Design review of the part built by this model. Coordinates are the model's own, in mm. A direction names the side the tool comes from. Coordinates: 2 decimals unless noted, no trailing zeros. Loops run counter-clockwise (first coordinate to the right, second up) from the corner with the lowest first, then second, coordinate; pieces in that order, holes last. Notation, with made-up numbers: (10, -0.75) -> (61, -0.75) arc R22 ccw to (61, 18.25) -> close; hole circle Ø11 at (-17, 78.5). An arc over 180 degrees is marked (long way). Answer in a Markdown table with one row per item.
```python
from build123d import *

# Parameters (mm, degrees)
F1_DEPTH = 628.65
F2_R     = 4.76249
F4_DEPTH = 25.4


# Not quite as in the source:
# - a fillet or chamfer is up to 0.001 mm smaller than in the source, because OpenCascade refuses the exact size


with BuildPart() as f1:
    # F0 (on Front) → F1 (new body)
    with BuildSketch(Plane.XZ):
        Polygon((0, 44.45), (0, 0), (44.45, 0), (44.45, 4.7625), (4.7625, 4.7625), (4.7625, 44.45), align=None)
    extrude(amount=F1_DEPTH)

    # F2 (radius 4.7625 in the source; OpenCascade refuses exactly that, so slightly less here)
    f2_edges = [f1.edges().sort_by_distance(p)[0] for p in [
        (4.7625, -314.325, 4.7625),
        (4.7625, -314.325, 44.45),
        (44.45, -314.325, 4.7625),
    ]]
    fillet(f2_edges, radius=F2_R)

    # F3 (on face) → F4 (cut)
    with BuildSketch(Plane(origin=(0, 0, 0), x_dir=(0, -1, 0), z_dir=(-1, 0, 0))):
        Polygon((0, 44.45), (0, 4.7625), (39.6875, 44.45), align=None)
        Polygon((628.65, 44.45), (532.8358992433, 44.45), (628.65, 4.7625), align=None)
    extrude(amount=-F4_DEPTH, mode=Mode.SUBTRACT)


solid = f1.part
```
(1) Tool access review of faces 1 (the flat face through (4.762, -307, 24)), 2 (the flat face through (2.579, -580.072, 24.884)): name each direction out of +Z, -Z, +X, -X, +Y, -Y from which nothing blocks a thin tool from reaching the whole face with its end or side.
Evaluation:
| item | result |
|---|---|
| face 1 | +Z, +X, +Y, -Y |
| face 2 | +Z, +X, -X, -Y |
(2) To check wall thickness, follow probe 1 along Z at (x, y) = (34, -210); probe 2 along Z at (x, y) = (2.5, -158.5). State the ranges of each line that lie inside material, in increasing order.
Evaluation:
| item | result |
|---|---|
| probe 1 | z = 0 to 4.76 |
| probe 2 | z = 0 to 43.74 |
(3) Take a section at C-C on z = 27. Give the boundary of the cut face in (x, y).
Evaluation:
| item | result |
|---|---|
| outline | (0, -574.96) -> (4.76, -574.96) -> (4.76, -22.24) -> (0, -22.24) -> close |
(4) Take a section at B-B on x = 31. Give the boundary of the cut face in (y, z), and give its area (3 significant figures).
Evaluation:
| item | result |
|---|---|
| outline | (-628.65, 0) -> (0, 0) -> (0, 4.76) -> (-628.65, 4.76) -> close |
| area | 2,990 mm² |
(5) For pin 1 (5 mm diameter, centred on x = 25, y = -81, fed in from +Z); pin 2 (5 mm diameter, centred on y = -139.5, z = 19.5, fed in from +X); pin 3 (5 mm diameter, centred on x = 9.5, y = -175, fed in from +Z), all flat-tipped, find the tip position at first contact; note any pin that passes through.
Evaluation:
| item | result |
|---|---|
| pin 1 | stops at z = 4.76 |
| pin 2 | stops at x = 4.76 |
| pin 3 | stops at z = 5.49 |
